Geometry check sheet. Reference: the model listing, model coordinates, mm. Face numbers are marked on the shaded views. A direction names the side the tool comes from. Give positions to 0.01 mm unless a question says otherwise; leave off trailing zeros. Loops run counter-clockwise (first coordinate to the right, second up) from the corner with the lowest first, then second, coordinate; pieces in that order, holes last. Notation, with made-up numbers: (40, 23.25) - (49, 23.25) arc R38 cw to (49, 62.25) - close; hole circle Ø7 at (85.5, 85.25). An arc over 180 degrees is marked (long way). Use a Markdown table: item, result. Add a question column.
1. Draft check along X on the marked faces 3, 4 and 5. Enter one of: pulls with the +X half, pulls with the -X half, needs draft (parallel to the pull), parting line crosses it, or undercut.
2. Cross-section at C-C on y = 62. Enter the section's corners in (x, z), and give its area (3 significant figures).
3. Depth check by flat-ended pin: P1, Ø12, axis at x = 1.5, z = 4, coming from the -Y side; P2, Ø8.5, axis at x = 0, z = 0, coming from the +Y side; P3, Ø10.5, axis at y = 10, z = 12, coming from the -X side; P4, Ø1.8, axis at x = -16.5, y = 14.5, coming from the -Z side. Enter the tip coordinate at first touch or a pass-through.
4. Material ranges on L1, parallel to X at y = 54.5, z = 8; L2, parallel to Y at x = 8, z = -8.5; L3, parallel to Z at x = -15.85, y = 10, recorded low to high.
5. Cross-section at B-B on z = 0. Enter the section's corners in (x, y), and give its area (3 significant figures).
6. Set-up check for the marked faces 1 and 2: record each of +Z, -Z, +X, -X, +Y, -Y from which the full face is reachable in a straight line by a thin tool's end or side.
7. Cross-section at D-D on y = 9. Enter the section's corners in (x, z), and give its area (3 significant figures).
8. Cross-section at A-A on x = 0. Enter the section's corners in (y, z).
from build123d import *

# Parameters (mm, degrees)
BASE_FLANGE1_DEPTH = 22
CUT_EXTRUDE2_START = -34.556
CUT_EXTRUDE2_DEPTH = 34.556
SKETCH9_R          = 4
CUT_EXTRUDE3_DEPTH = 82.345647825
SKETCH10_R         = 7.25
CUT_EXTRUDE4_DEPTH = 76.640773185
CUT_EXTRUDE5_REACH = 83.346


# Read off the part's stored shape, not the designer's step: Cut-Extrude2
# Sheet-metal steps are written as plain solids
with BuildPart() as part:
    # Sketch2 → Base-Flange1 (new, symmetric)
    with BuildSketch(Plane.XY):
        with BuildLine():
            Line((15, 0), (15, 65))
            ThreePointArc((15, 65), (14.121320344, 67.121320344), (12, 68))
            Line((12, 68), (-12, 68))
            ThreePointArc((-12, 68), (-14.121320344, 67.121320344), (-15, 65))
            Line((-15, 65), (-15, 0))
            Line((-15, 0), (-17.278, 0))
            Line((-17.278, 0), (-17.278, 65))
            ThreePointArc((-17.278, 65), (-15.732109591, 68.732109591), (-12, 70.278))
            Line((-12, 70.278), (12, 70.278))
            ThreePointArc((12, 70.278), (15.732109591, 68.732109591), (17.278, 65))
            Line((17.278, 65), (17.278, 0))
            Line((17.278, 0), (15, 0))
        make_face()
    extrude(amount=BASE_FLANGE1_DEPTH, both=True)

    # Cut-Extrude2 outline → Cut-Extrude2 (cut)
    with BuildSketch(Plane(origin=(17.278, 0, 0), x_dir=(0, 0, -1), z_dir=(1, 0, 0)).offset(CUT_EXTRUDE2_START)):
        with BuildLine():
            Line((22, 65), (-2.783188769, 6.120516693))
            ThreePointArc((-2.783188769, 6.120516693), (-6.468039819, 1.669488818), (-12.000000004, 0))
            Line((-12.000000004, 0), (22, 0))
            Line((22, 0), (22, 65))
        make_face()
        with BuildLine():
            Line((-22, 0), (-12.000000004, 0))
            ThreePointArc((-12.000000004, 0), (-19.071067813, 2.92893219), (-22, 10))
            Line((-22, 10), (-22, 0))
        make_face()
    extrude(amount=CUT_EXTRUDE2_DEPTH, mode=Mode.SUBTRACT)

    # Sketch9 → Cut-Extrude3 (cut, through all)
    with BuildSketch(Plane(origin=(17.278, 0, 0), x_dir=(0, 0, -1), z_dir=(1, 0, 0))):
        with Locations((-12, 10)):
            Circle(SKETCH9_R)
    extrude(amount=-CUT_EXTRUDE3_DEPTH, mode=Mode.SUBTRACT)

    # Sketch10 → Cut-Extrude4 (cut, through all)
    with BuildSketch(Plane(origin=(0, 70.278, 0), x_dir=(1, 0, 0), z_dir=(0, 1, 0))):
        with Locations(Location((0, 0, 0), (0, 0, 270))):
            Circle(SKETCH10_R)
    extrude(amount=-CUT_EXTRUDE4_DEPTH, mode=Mode.SUBTRACT)

    # Sketch13 → Cut-Extrude5 (cut, up to next)
    with BuildSketch(Plane.ZY.offset(17.278), mode=Mode.PRIVATE) as cut_extrude5_sk1:
        with BuildLine():
            ThreePointArc((10.75, 13.799671038), (12, 14), (13.25, 13.799671038))
            Line((13.25, 13.799671038), (13.25, 16))
            Line((13.25, 16), (10.75, 16))
            Line((10.75, 16), (10.75, 13.799671038))
        make_face()
    cut_extrude5_tool1 = extrude(cut_extrude5_sk1.sketch, amount=-CUT_EXTRUDE5_REACH, mode=Mode.PRIVATE) & part.part
    add(cut_extrude5_tool1.solids().sort_by_distance((-17.278, 14.966097, 12))[0], mode=Mode.SUBTRACT)


solid = part.part
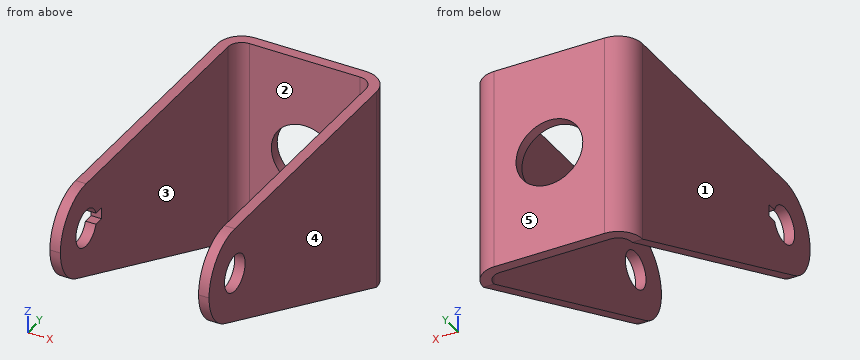
Values found:
| question | item | result |
|---|---|---|
| 1 | face 3 | undercut |
| 1 | face 4 | pulls with the +X half |
| 1 | face 5 | needs draft |
| 2 | outline | (-17.28, -20.74) - (-15, -20.74) - (-15, 22) - (-17.28, 22) - close; (15, -20.74) - (17.28, -20.74) - (17.28, 22) - (15, 22) - close |
| 2 | area | 195 mm2 |
| 3 | P1 | stops at y = 68 |
| 3 | P2 | passes through |
| 3 | P3 | stops at x = -17.28 |
| 3 | P4 | stops at z = -1.12 |
| 4 | L1 | x = -17.28 to -15, 15 to 17.28 |
| 4 | L2 | y = 68 to 70.28 |
| 4 | L3 | z = 1.15 to 8, 16 to 22 |
| 5 | outline | (-17.28, 12.73) - (-15, 12.73) - (-15, 65) arc R3 cw to (-12, 68) - (-7.25, 68) - (-7.25, 70.28) - (-12, 70.28) arc R5.28 ccw to (-17.28, 65) - close; (7.25, 68) - (12, 68) arc R3 cw to (15, 65) - (15, 12.73) - (17.28, 12.73) - (17.28, 65) arc R5.28 ccw to (12, 70.28) - (7.25, 70.28) - close |
| 5 | area | 289 mm2 |
| 6 | face 1 | +Z, -Z, -X, +Y, -Y |
| 6 | face 2 | +Z, -Z, -Y |
| 7 | outline | (-17.28, 1.57) - (-15, 1.57) - (-15, 8.13) - (-17.28, 8.13) - close; (-17.28, 15.87) - (-15, 15.87) - (-15, 21.95) - (-17.28, 21.95) - close; (15, 1.57) - (17.28, 1.57) - (17.28, 8.13) - (15, 8.13) - close; (15, 15.87) - (17.28, 15.87) - (17.28, 21.95) - (15, 21.95) - close |
| 7 | area | 57.6 mm2 |
| 8 | outline | (68, -22) - (70.28, -22) - (70.28, -7.25) - (68, -7.25) - close; (68, 7.25) - (70.28, 7.25) - (70.28, 22) - (68, 22) - close |
